Source: CAD feature listing. Evaluate the final solid. Frame: model axes, mm. Face numbers are marked on the shaded views. A direction names the side the tool comes from. Give positions to 0.01 mm unless a question says otherwise; leave off trailing zeros. Loops run counter-clockwise (first coordinate to the right, second up) from the corner with the lowest first, then second, coordinate; pieces in that order, holes last. Notation, with made-up numbers: (5.5, -8.75) - (35.5, -8.75) arc R19 cw to (35.5, 27.25) - close; hole circle Ø5 at (86, 87.5). An arc over 180 degrees is marked (long way). Write each question's results on one line, items separated by ' | '. Start each with the question number.
(1) Pull-direction query (Z, two-part tool) for the marked faces 6, 7, 8 and 9; classes: pulls with the +Z half, pulls with the -Z half, needs draft (parallel to the pull), parting line crosses it, or undercut.
(2) Material intervals for line 1 along X through (y, z) = (10, -23); line 2 along Z through (x, y) = (113.5, 12.5); line 3 along Z through (x, y) = (75, 31), sorted ascending. Write a range as [from, to].
(3) Cut plane A-A on z = -158.5. Return the cut outline in (x, y).
(4) Cut plane C-C on x = 131. Return the cut outline in (y, z), then the cut area to 3 significant figures.
(5) Contact query for flat-ended pins moving along their axis: pin 1 (15 mm diameter, centred on x = 164.5, z = -160.5, fed in from +Y); pin 2 (12.5 mm diameter, centred on x = 161.5, y = 11.5, fed in from +Z); pin 3 (14 mm diameter, centred on x = 70.5, y = 33.5, fed in from +Z). Output: stop coordinate, or through.
(6) Reachability of the marked faces 1, 2, 3, 4 and 5 from +Z, -Z, +X, -X, +Y, -Y: full face, straight path, thin tool, end or side. Return the list, or none.
(7) Cut plane D-D on z = -120.65. Return the cut outline in (x, y).
(8) Cut plane B-B on y = 10. Return the cut outline in (x, z).
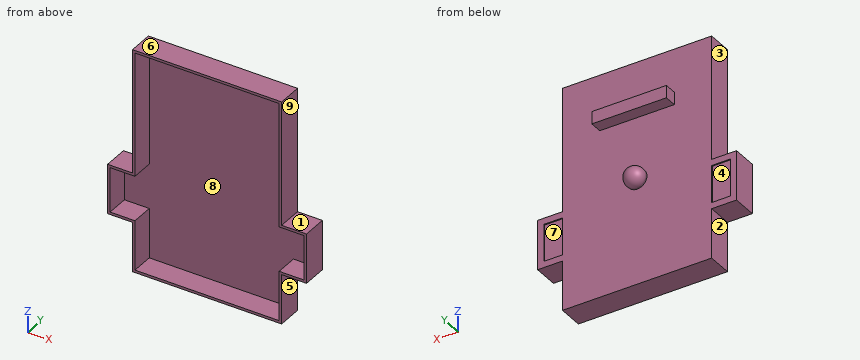
from build123d import *

# Parameters (mm, degrees)
SKETCH1_W           = 152.4
SKETCH1_H           = 228.6
BOSS_EXTRUDE1_DEPTH = 25.4
SKETCH5_W           = 25.4
SKETCH5_H           = 50.8
BOSS_EXTRUDE5_DEPTH = 25.4
SHELL1_T            = -2.54
SKETCH4_W           = 76.2
SKETCH4_H           = 12.7
BOSS_EXTRUDE4_DEPTH = 12.7
SKETCH3_R           = 10.121060994
BOSS_EXTRUDE3_DEPTH = 1.27
DOME1_FACE_RADIUS   = 10.121060994
DOME1_HEIGHT        = 12.7
SKETCH7_W           = 19.05
SKETCH7_H           = 38.1
CUT_EXTRUDE1_DEPTH  = 1.27


with BuildPart() as part:
    # Sketch1 → Boss-Extrude1 (new body)
    with BuildSketch(Plane(origin=(0, 0, 0), x_dir=(1, 0, 0), z_dir=(0, 1, 0))):
        with Locations((76.2, 114.3)):
            Rectangle(SKETCH1_W, SKETCH1_H)
    extrude(amount=BOSS_EXTRUDE1_DEPTH)

    # Sketch5 → Boss-Extrude5 (add)
    with BuildSketch(Plane(origin=(0, 25.4, 0), x_dir=(1, 0, 0), z_dir=(0, 1, 0))):
        with Locations((165.1, 152.4)):
            Rectangle(SKETCH5_W, SKETCH5_H)
        with Locations((-12.7, 152.4)):
            Rectangle(SKETCH5_W, SKETCH5_H)
    extrude(amount=-BOSS_EXTRUDE5_DEPTH)

    # Shell1
    shell1_openings = [part.faces().sort_by_distance(p)[0] for p in [
        (76.2, 0, -116.927586207),
    ]]
    offset(amount=SHELL1_T, openings=shell1_openings, kind=Kind.INTERSECTION)

    # Sketch4 → Boss-Extrude4 (add)
    with BuildSketch(Plane(origin=(0, 25.4, 0), x_dir=(1, 0, 0), z_dir=(0, 1, 0))):
        with Locations((76.2, 50.8)):
            Rectangle(SKETCH4_W, SKETCH4_H)
    extrude(amount=BOSS_EXTRUDE4_DEPTH)

    # Sketch3 → Boss-Extrude3 (add)
    with BuildSketch(Plane(origin=(0, 25.4, 0), x_dir=(1, 0, 0), z_dir=(0, 1, 0))):
        with Locations(Location((76.2, 120.65, 0), (0, 0, 90))):
            Circle(SKETCH3_R)
    extrude(amount=BOSS_EXTRUDE3_DEPTH)

    # Dome1: a dome of height H over a round flat face of radius A is a cap of a sphere of radius (A * A + H * H) / (2 * H)
    dome1_r = (DOME1_FACE_RADIUS * DOME1_FACE_RADIUS + DOME1_HEIGHT * DOME1_HEIGHT) / (2 * DOME1_HEIGHT)
    dome1_base = Plane((76.2, 26.67, -120.65), z_dir=(0, 1, 0))
    with Locations(dome1_base.offset(DOME1_HEIGHT - dome1_r)):
        dome1_ball = Sphere(dome1_r, mode=Mode.PRIVATE)
    add(split(dome1_ball, bisect_by=dome1_base, keep=Keep.TOP, mode=Mode.PRIVATE))

    # Sketch7 → Cut-Extrude1 (cut)
    with BuildSketch(Plane(origin=(0, 25.4, 0), x_dir=(1, 0, 0), z_dir=(0, 1, 0))):
        with Locations((-9.525, 152.4)):
            Rectangle(SKETCH7_W, SKETCH7_H)
        with Locations((161.925, 152.4)):
            Rectangle(SKETCH7_W, SKETCH7_H)
    extrude(amount=-CUT_EXTRUDE1_DEPTH, mode=Mode.SUBTRACT)


solid = part.part
Ans:
1) face 6: pulls with the +Z half | face 7: undercut | face 8: undercut | face 9: needs draft
2) line 1: [0, 2.54], [149.86, 152.4] | line 2: [-228.6, -226.06], [-2.54, 0] | line 3: [-130.76, -110.54], [-57.15, -44.45]
3) outline: (-25.4, 0) - (-22.86, 0) - (-22.86, 22.86) - (175.26, 22.86) - (175.26, 0) - (177.8, 0) - (177.8, 25.4) - (171.45, 25.4) - (171.45, 24.13) - (152.4, 24.13) - (152.4, 25.4) - (0, 25.4) - (0, 24.13) - (-19.05, 24.13) - (-19.05, 25.4) - (-25.4, 25.4) - close
4) outline: (0, -228.6) - (25.4, -228.6) - (25.4, 0) - (0, 0) - (0, -2.54) - (22.86, -2.54) - (22.86, -226.06) - (0, -226.06) - close | area: 697 mm^2
5) pin 1: y = 25.4 | pin 2: z = -127 | pin 3: z = -44.45
6) face 1: +Z, +X, +Y, -Y | face 2: -Z, -X, +Y, -Y | face 3: +Z, -X, +Y, -Y | face 4: +Y | face 5: -Z, +X, +Y, -Y
7) outline: (0, 0) - (2.54, 0) - (2.54, 22.86) - (149.86, 22.86) - (149.86, 0) - (152.4, 0) - (152.4, 25.4) - (86.32, 25.4) - (86.32, 26.67) arc R10.38 ccw (long way) to (66.08, 26.67) - (66.08, 25.4) - (0, 25.4) - close
8) outline: (-25.4, -177.8) - (0, -177.8) - (0, -228.6) - (152.4, -228.6) - (152.4, -177.8) - (177.8, -177.8) - (177.8, -127) - (152.4, -127) - (152.4, 0) - (0, 0) - (0, -127) - (-25.4, -127) - close; hole (-22.86, -175.26) - (2.54, -175.26) - (2.54, -226.06) - (149.86, -226.06) - (149.86, -175.26) - (175.26, -175.26) - (175.26, -129.54) - (149.86, -129.54) - (149.86, -2.54) - (2.54, -2.54) - (2.54, -129.54) - (-22.86, -129.54) - close
